Geometry check sheet. Reference: the model listing, model coordinates, mm. Give positions to 0.01 mm unless a question says otherwise; leave off trailing zeros. One line per item, written item: value. Start each with the question number.
1. Cross-section at A-A on z = -39.05. Count the separate pieces of the cut face and the enclosed holes in it, then the cut area to 3 significant figures.
2. Release check for a two-part mould opening along Y. For faces 1 (the face through (0, 0, -39.592)), 2 (the face through (8.91, -4.35, -39.19)) record: pulls with the +Y half, pulls with the -Y half, needs draft (parallel to the pull), parting line crosses it, or undercut.
3. Scan lines: line 1 (X direction, y = -5.75, z = -39); line 2 (X direction, y = -1.75, z = -38.95); line 3 (X direction, y = -3, z = -39.15). Record each from-to range of solid material in increasing order.
4. Gauge pin test, flat end, axial feed: pin 1 (1.4 mm diameter, centred on x = -8.255, y = -4.953, fed in from -Z). Record the tip position at first contact, or that the pin passes through.
from build123d import *

# Parameters (mm, degrees)
BOSS_EXTRUDE1_DEPTH     = 0.8
SKETCH2_R               = 0.3556
CUT_EXTRUDE1_DEPTH      = 27.149953829
CUT_EXTRUDE2_DEPTH      = 27.149953829
CUT_EXTRUDE2_DEPTH_BACK = 27.149953829
SKETCH3_R               = 0.889


with BuildPart() as part:
    # Sketch1 → Boss-Extrude1 (new body)
    with BuildSketch(Plane(origin=(0, 0, -38.7925), x_dir=(-1, 0, 0), z_dir=(0, 0, -1))):
        with BuildLine():
            Line((23.8125, 6.6675), (-23.8125, 6.6675))
            ThreePointArc((-23.8125, 6.6675), (-25.272010309, 5.153242143), (-23.705057143, 3.750457422))
            ThreePointArc((-23.705057143, 3.750457422), (-23.130382387, 3.548805041), (-22.887, 2.990522163))
            Line((-22.887, 2.990522163), (-22.887, -2.990522163))
            ThreePointArc((-22.887, -2.990522163), (-23.130382387, -3.548805041), (-23.705057143, -3.750457422))
            ThreePointArc((-23.705057143, -3.750457422), (-25.272010309, -5.153242143), (-23.8125, -6.6675))
            Line((-23.8125, -6.6675), (23.8125, -6.6675))
            ThreePointArc((23.8125, -6.6675), (25.272010309, -5.153242143), (23.705057143, -3.750457422))
            ThreePointArc((23.705057143, -3.750457422), (23.130382387, -3.548805041), (22.887, -2.990522163))
            Line((22.887, -2.990522163), (22.887, 2.990522163))
            ThreePointArc((22.887, 2.990522163), (23.130382387, 3.548805041), (23.705057143, 3.750457422))
            ThreePointArc((23.705057143, 3.750457422), (25.272010309, 5.153242143), (23.8125, 6.6675))
        make_face()
    extrude(amount=BOSS_EXTRUDE1_DEPTH)

    # Sketch2 → Cut-Extrude1 (cut, through all)
    with BuildSketch(Plane(origin=(0, 0, -39.5925), x_dir=(-1, 0, 0), z_dir=(0, 0, -1))):
        with Locations((-7.62, -1.905)):
            Circle(SKETCH2_R)
        with Locations((-8.89, -1.905)):
            Circle(SKETCH2_R)
        with Locations((-7.62, 1.905)):
            Circle(SKETCH2_R)
        with Locations((-8.89, 1.905)):
            Circle(SKETCH2_R)
        with Locations((-7.62, 0.635)):
            Circle(SKETCH2_R)
        with Locations((-8.89, 0.635)):
            Circle(SKETCH2_R)
        with Locations((-7.62, -0.635)):
            Circle(SKETCH2_R)
        with Locations((-8.89, -0.635)):
            Circle(SKETCH2_R)
        with Locations((8.89, 1.905)):
            Circle(SKETCH2_R)
        with Locations((7.62, 1.905)):
            Circle(SKETCH2_R)
        with Locations((8.89, -1.905)):
            Circle(SKETCH2_R)
        with Locations((7.62, -1.905)):
            Circle(SKETCH2_R)
        with Locations((8.89, -0.635)):
            Circle(SKETCH2_R)
        with Locations((7.62, -0.635)):
            Circle(SKETCH2_R)
        with Locations((8.89, 0.635)):
            Circle(SKETCH2_R)
        with Locations((7.62, 0.635)):
            Circle(SKETCH2_R)
    extrude(amount=-CUT_EXTRUDE1_DEPTH, mode=Mode.SUBTRACT)

    # Sketch3 → Cut-Extrude2 (cut, two sides: drawn at the far end of the back side and taken through both)
    with BuildSketch(Plane(origin=(0, 0, -39.5925), x_dir=(-1, 0, 0), z_dir=(0, 0, -1)).offset(-CUT_EXTRUDE2_DEPTH_BACK)):
        with Locations((-23.8125, 5.207)):
            Circle(SKETCH3_R)
        with Locations((-23.8125, -5.207)):
            Circle(SKETCH3_R)
        with Locations((23.8125, 5.207)):
            Circle(SKETCH3_R)
        with Locations((23.8125, -5.207)):
            Circle(SKETCH3_R)
        with Locations((-8.255, 4.953)):
            Circle(SKETCH3_R)
        with Locations((8.255, 4.953)):
            Circle(SKETCH3_R)
        with Locations((8.255, -4.953)):
            Circle(SKETCH3_R)
        with Locations((-8.255, -4.953)):
            Circle(SKETCH3_R)
    extrude(amount=CUT_EXTRUDE2_DEPTH + CUT_EXTRUDE2_DEPTH_BACK, mode=Mode.SUBTRACT)


solid = part.part
Report:
1. separate pieces: 1
1. enclosed holes: 24
1. area: 609 mm^2
2. face 1: needs draft
2. face 2: undercut
3. line 1: x = -25.17 to -24.52, -23.11 to -8.65, -7.86 to 7.86, 8.65 to 23.11, 24.52 to 25.17
3. line 2: x = -22.89 to -9.21, -8.57 to -7.94, -7.3 to 7.3, 7.94 to 8.57, 9.21 to 22.89
3. line 3: x = -22.89 to 22.89
4. pin 1: passes through
